Study the drawing (mm; zero at the part's minimum x, y, z) and answer. A direction names the side the tool comes from. Coordinates: 2 decimals unless noted, no trailing zeros. Order: outer loops, then holes, each group sorted by start corner. A loop starts at its lowest first (then second) coordinate and runs counter-clockwise, first axis right, second up. Notation, with made-up numbers: (65.25, 85.5) -> (110.25, 85.5) arc R14 ccw to (110.25, 97.5) -> close; hole circle Ø11 at (-6, 3.5). An arc over 180 degrees is marked (long way). Write each question's results on one line, items separated by ' | '. Start each with the question number.
(1) Given pin 1 (5 mm diameter, centred on x = 52.5, y = 8, fed in from +Z); pin 2 (11.5 mm diameter, centred on x = 30, z = 25, fed in from -Y); pin 3 (12 mm diameter, centred on x = 53.5, y = 10, fed in from +Z), each flat-ended and moving along its own axis, determine where each tip first touches the part or whether it passes through.
(2) Determine the mould class of the marked faces 1, 2 and 3 for opening direction X: +X half, -X half, draft (parallel to the pull), parting line (faces both ways), or undercut.
(3) The part is cut by section D-D, the plane x = 53. Give the vertices of the cut face in (y, z).
(4) The part is cut by section B-B, the plane x = 30. Give the vertices of the cut face in (y, z), then the cut area to 3 significant figures.
(5) The part is cut by section C-C, the plane z = 25. Count the separate pieces of the cut face and the enclosed holes in it, then the cut area to 3 significant figures.
(6) A tool of negligible diameter and unlimited length cuts with its end or side. For the marked faces 4, 5 and 6, from which of +Z, -Z, +X, -X, +Y, -Y can it reach the whole face along a straight path? Write none if from no direction.
(7) The part is cut by section A-A, the plane y = 10. Give the vertices of the cut face in (x, z).
(8) Straight lines are drawn through the part: L1, parallel to Z at x = 53, y = 5.25; L2, parallel to Z at x = 53, y = 3.75; L3, parallel to X at y = 5, z = 8.5. For each, find the intervals that lie inside material, in ascending order.
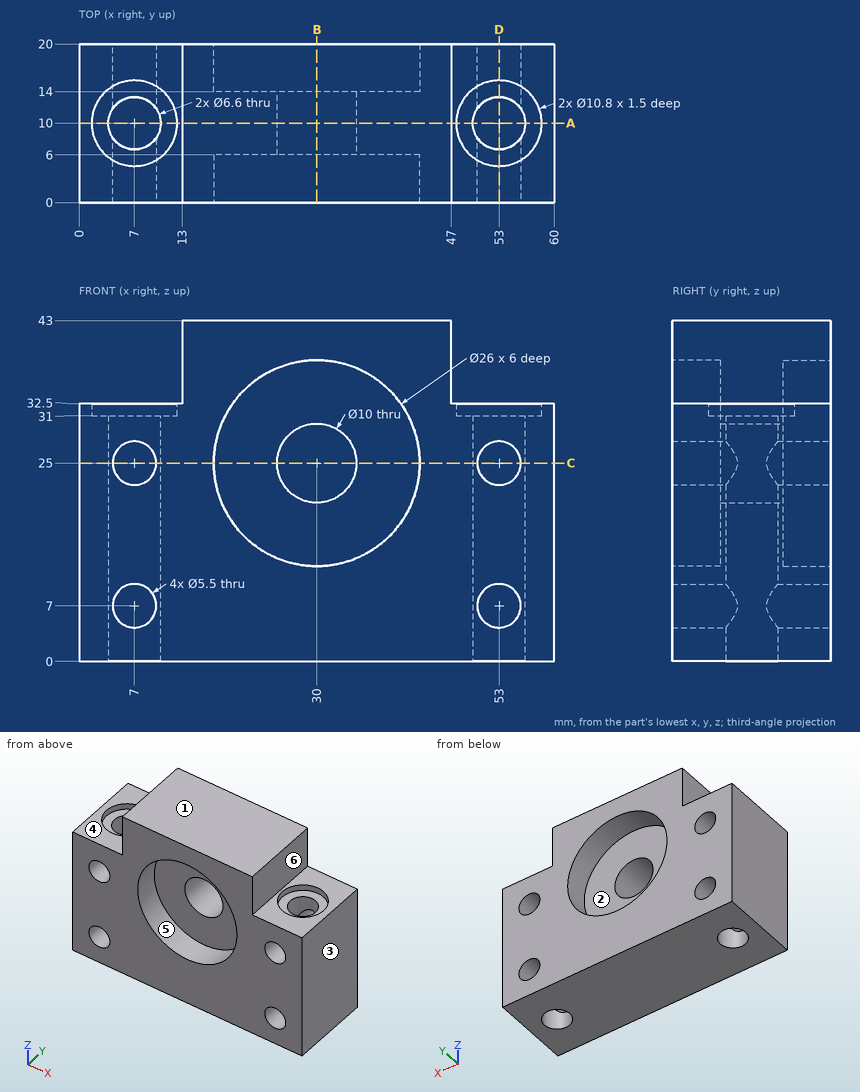
Established:
1) pin 1: stops at z = 31 | pin 2: stops at y = 6 | pin 3: stops at z = 32.5
2) face 1: draft | face 2: undercut | face 3: +X half
3) outline: (0, 0) -> (6.7, 0) -> (6.7, 4.25) -> (0, 4.25) -> close; (0, 9.75) -> (6.7, 9.75) -> (6.7, 22.25) -> (0, 22.25) -> close; (0, 27.75) -> (6.7, 27.75) -> (6.7, 31) -> (4.6, 31) -> (4.6, 32.5) -> (0, 32.5) -> close; (13.3, 0) -> (20, 0) -> (20, 4.25) -> (13.3, 4.25) -> close; (13.3, 9.75) -> (20, 9.75) -> (20, 22.25) -> (13.3, 22.25) -> close; (13.3, 27.75) -> (20, 27.75) -> (20, 32.5) -> (15.4, 32.5) -> (15.4, 31) -> (13.3, 31) -> close
4) outline: (0, 0) -> (20, 0) -> (20, 12) -> (14, 12) -> (14, 20) -> (6, 20) -> (6, 12) -> (0, 12) -> close; (0, 38) -> (6, 38) -> (6, 30) -> (14, 30) -> (14, 38) -> (20, 38) -> (20, 43) -> (0, 43) -> close | area: 468 mm^2
5) separate pieces: 4 | enclosed holes: 0 | area: 583 mm^2
6) face 4: +Z, -X, +Y, -Y | face 5: -Y | face 6: +Z, +X, +Y, -Y
7) outline: (0, 0) -> (3.7, 0) -> (3.7, 31) -> (1.6, 31) -> (1.6, 32.5) -> (0, 32.5) -> close; (10.3, 0) -> (49.7, 0) -> (49.7, 31) -> (47.6, 31) -> (47.6, 32.5) -> (47, 32.5) -> (47, 43) -> (13, 43) -> (13, 32.5) -> (12.4, 32.5) -> (12.4, 31) -> (10.3, 31) -> close; (56.3, 0) -> (60, 0) -> (60, 32.5) -> (58.4, 32.5) -> (58.4, 31) -> (56.3, 31) -> close; hole circle Ø10 at (30, 25)
8) L1: z = 0 to 4.25, 9.75 to 22.25, 27.75 to 31 | L2: z = 0 to 4.25, 9.75 to 22.25, 27.75 to 32.5 | L3: x = 0 to 4.7, 9.3 to 50.7, 55.3 to 60
